For this review, take the finished solid that the model builds, in its own axes (mm). Round coordinates to 2 decimals unless told otherwise and drop trailing zeros. Order: outer loops, then holes, each group sorted by start corner. A loop starts at its lowest first (then second) coordinate and runs counter-clockwise, first axis right, second up.
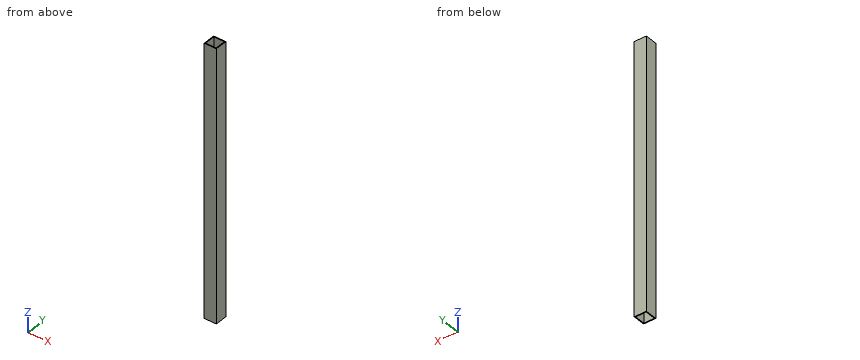
from build123d import *

# Parameters (mm, degrees)
CROQUIS2_W              = 76.2
CROQUIS2_H              = 76.2
CROQUIS2_W_2            = 66.675
CROQUIS2_H_2            = 66.675
SALIENTE_EXTRUIR1_DEPTH = 1700


with BuildPart() as part:
    # Croquis2 → Saliente-Extruir1 (new body)
    with BuildSketch(Plane.XY):
        with Locations((38.1, -38.1)):
            Rectangle(CROQUIS2_W, CROQUIS2_H)
        with Locations((38.1, -38.1)):
            Rectangle(CROQUIS2_W_2, CROQUIS2_H_2, mode=Mode.SUBTRACT)
    extrude(amount=-SALIENTE_EXTRUIR1_DEPTH)


solid = part.part
(1) Add section B-B on y = -31. Give the boundary of the cut face in (x, z).
(2) Add section C-C on z = -653. Give the boundary of the cut face in (x, y), plus the area to 3 significant figures.
(3) Wall thickness on L1, parallel to Y at x = 17, z = -1463.5; L2, parallel to X at y = -25.5, z = -639.5: over which ranges is each line inside the solid? List them lowest first.
(4) Add section A-A on x = 48. Give the boundary of the cut face in (y, z), plus the area to 3 significant figures.
Here are the results:
1. outline: (0, -1700) - (4.76, -1700) - (4.76, 0) - (0, 0) - close; (71.44, -1700) - (76.2, -1700) - (76.2, 0) - (71.44, 0) - close
2. outline: (0, -76.2) - (76.2, -76.2) - (76.2, 0) - (0, 0) - close; hole (4.76, -71.44) - (71.44, -71.44) - (71.44, -4.76) - (4.76, -4.76) - close
2. area: 1,360 mm2
3. L1: y = -76.2 to -71.44, -4.76 to 0
3. L2: x = 0 to 4.76, 71.44 to 76.2
4. outline: (-76.2, -1700) - (-71.44, -1700) - (-71.44, 0) - (-76.2, 0) - close; (-4.76, -1700) - (0, -1700) - (0, 0) - (-4.76, 0) - close
4. area: 16,200 mm2
